from build123d import *

# Parameters (mm, degrees)
F1_DEPTH = 15
F2_DEPTH = 3
F0_W     = 146
F0_H     = 3
F3_DEPTH = 3
F0_W_2   = 20
F0_H_2   = 8
F4_DEPTH = 25
F5_R     = 6.5
F6_DEPTH = 11.3693
F7_R     = 3.99999


# Not quite as in the source:
# - a fillet or chamfer is up to 0.001 mm smaller than in the source, because OpenCascade refuses the exact size


with BuildPart() as f1:
    # F0 (on Top) → F1 (new body)
    with BuildSketch(Plane.XY):
        Polygon((-21.6026537657, 32.1407727134), (-91.6026537657, 32.1407727134), (-91.6026537657, -50.4549115884), (-81.6026537657, -50.8592272866), (-81.6026537657, -47.8592272866), (-84.6026537657, -47.8592272866), (-86.6026537657, -47.8592272866), (-86.6026537657, 27.1407727134), (-84.6026537657, 27.1407727134), (61.3973462343, 27.1407727134), (63.3973462343, 27.1407727134), (63.3973462343, -47.8592272866), (61.3973462343, -47.8592272866), (58.3973462343, -47.8592272866), (58.3973462343, -50.8592272866), (68.3973462343, -50.8592272866), (68.3973462343, 32.1407727134), (-1.6026537657, 32.1407727134), align=None)
    extrude(amount=F1_DEPTH)

    # F0 (on Top) → F2 (join)
    with BuildSketch(Plane.XY):
        Polygon((-86.6026537657, -47.8592272866), (-84.6026537657, -47.8592272866), (-84.6026537657, 24.1407727134), (-84.6026537657, 27.1407727134), (-86.6026537657, 27.1407727134), align=None)
        Polygon((61.3973462343, 27.1407727134), (61.3973462343, 24.1407727134), (61.3973462343, -47.8592272866), (63.3973462343, -47.8592272866), (63.3973462343, 27.1407727134), align=None)
    extrude(amount=F2_DEPTH)

    # F0 (on Top) → F3 (join)
    with BuildSketch(Plane.XY):
        with Locations((-11.6026537657, 25.6407727134)):
            Rectangle(F0_W, F0_H)
    extrude(amount=F3_DEPTH)

    # F0 (on Top) → F4 (join)
    with BuildSketch(Plane.XY):
        with Locations((-11.6026537657, 36.1407727134)):
            Rectangle(F0_W_2, F0_H_2)
    extrude(amount=F4_DEPTH)

    # F5 (on Right) → F6 (cut)
    with BuildSketch(Plane.YZ):
        with Locations((36.1407727134, 20)):
            Circle(F5_R)
        Polygon((33.2721245414, 20.362976629), (34.0333399009, 21.979803351), (35.5995229657, 22.8404124839), (37.3724450378, 22.61608059), (38.674910145, 21.3924948281), (39.0094208855, 19.637023371), (38.248205526, 18.020196649), (36.6820224612, 17.1595875161), (34.9091003891, 17.38391941), (33.6066352819, 18.6075051719), align=None, mode=Mode.SUBTRACT)
    extrude(amount=-F6_DEPTH, mode=Mode.SUBTRACT)

    # F7 (radius 4 in the source; OpenCascade refuses exactly that, so slightly less here)
    f7_edges = [f1.edges().sort_by_distance(p)[0] for p in [
        (-16.485977, 40.140773, 25),
        (-16.485977, 32.140773, 25),
    ]]
    fillet(f7_edges, radius=F7_R)


solid = f1.part
Can you work these out from the model? Positions are in its coordinate system, mm. A direction names the side the tool comes from. Give positions to 0.01 mm unless a question says otherwise; leave off trailing zeros. Order: outer loops, then holes, each group sorted by start corner. A loop starts at its lowest first (then second) coordinate and runs counter-clockwise, first axis right, second up. Notation, with made-up numbers: M 26.5,-16.75 L 69.5,-16.75 A21 ccw 69.5,-4.75 Z; hole C 9,72 d10. An arc over 180 degrees is marked long. Use a Markdown table: item, result. Add a question column.
Item 1: If I drill on L1, parallel to X at y = -13, z = 3.75; L2, parallel to X at y = 17.5, z = 2.75; L3, parallel to Y at x = 14.5, z = 4, over which ranges is the centre line in solid material (lowest first)? Write a range as [from, to].
Item 2: For faces 5 (the flat face through (-81.603, -49, 7)), 6 (the flat face through (-1.603, 36, 7)), 7 (the flat face through (-86.603, -11, 9)), which set-ups out of +Z, -Z, +X, -X, +Y, -Y let a thin tool reach every point of the face, with its end or its side?
Item 3: Will these pins go through, and if not, where does the flat tip stop? pin 1 (5 mm diameter, centred on x = -41, z = 6, fed in from +Y); pin 2 (13 mm diameter, centred on x = -40, z = 10.5, fed in from -Y); pin 3 (4 mm diameter, centred on y = 36, z = 21.5, fed in from +X); pin 4 (2 mm diameter, centred on x = -43, z = 17, fed in from +Y).
Item 4: Suppose I cut it at A-A (y = -15.5). List the corners of the cut face in (x, z) for me, then the cut area to 3 significant figures.
Item 5: We'd pull the mould along Y, two halves only. Please class faces 1 (the flat face through (63.397, -10, 9)), 2 (the flat face through (68.397, -10, 7)), 3 (the flat face through (-84, -47.859, 7)), 4 (the flat face through (-17, 32.141, 18)): +Y half, -Y half, draft (parallel to the pull), parting line (faces both ways), or undercut.
Item 6: Suppose I cut it at C-C (z = 6.25). List the corners of the cut face in (x, y) for me, then the cut area to 3 significant figures.
Item 7: Suppose I cut it at B-B (x = -47). List the corners of the cut face in (y, z) for me, then the cut area to 3 significant figures.
Answer sheet:
| question | item | result |
|---|---|---|
| 1 | L1 | x = [-91.6, -86.6], [63.4, 68.4] |
| 1 | L2 | x = [-91.6, -84.6], [61.4, 68.4] |
| 1 | L3 | y = [27.14, 32.14] |
| 2 | face 5 | +Z, -Z, -Y |
| 2 | face 6 | +Z, -Z, +X, +Y |
| 2 | face 7 | +Z |
| 3 | pin 1 | stops at y = 32.14 |
| 3 | pin 2 | stops at y = 27.14 |
| 3 | pin 3 | stops at x = -1.6 |
| 3 | pin 4 | passes through |
| 4 | outline | M -91.6,0 L -84.6,0 L -84.6,3 L -86.6,3 L -86.6,15 L -91.6,15 Z; M 61.4,0 L 68.4,0 L 68.4,15 L 63.4,15 L 63.4,3 L 61.4,3 Z |
| 4 | area | 162 mm² |
| 5 | face 1 | undercut |
| 5 | face 2 | draft |
| 5 | face 3 | undercut |
| 5 | face 4 | -Y half |
| 6 | outline | M -91.6,-50.45 L -81.6,-50.86 L -81.6,-47.86 L -86.6,-47.86 L -86.6,27.14 L 63.4,27.14 L 63.4,-47.86 L 58.4,-47.86 L 58.4,-50.86 L 68.4,-50.86 L 68.4,32.14 L -1.6,32.14 L -1.6,40.14 L -21.6,40.14 L -21.6,32.14 L -91.6,32.14 Z |
| 6 | area | 1,770 mm² |
| 7 | outline | M 24.14,0 L 32.14,0 L 32.14,15 L 27.14,15 L 27.14,3 L 24.14,3 Z |
| 7 | area | 84.0 mm² |
